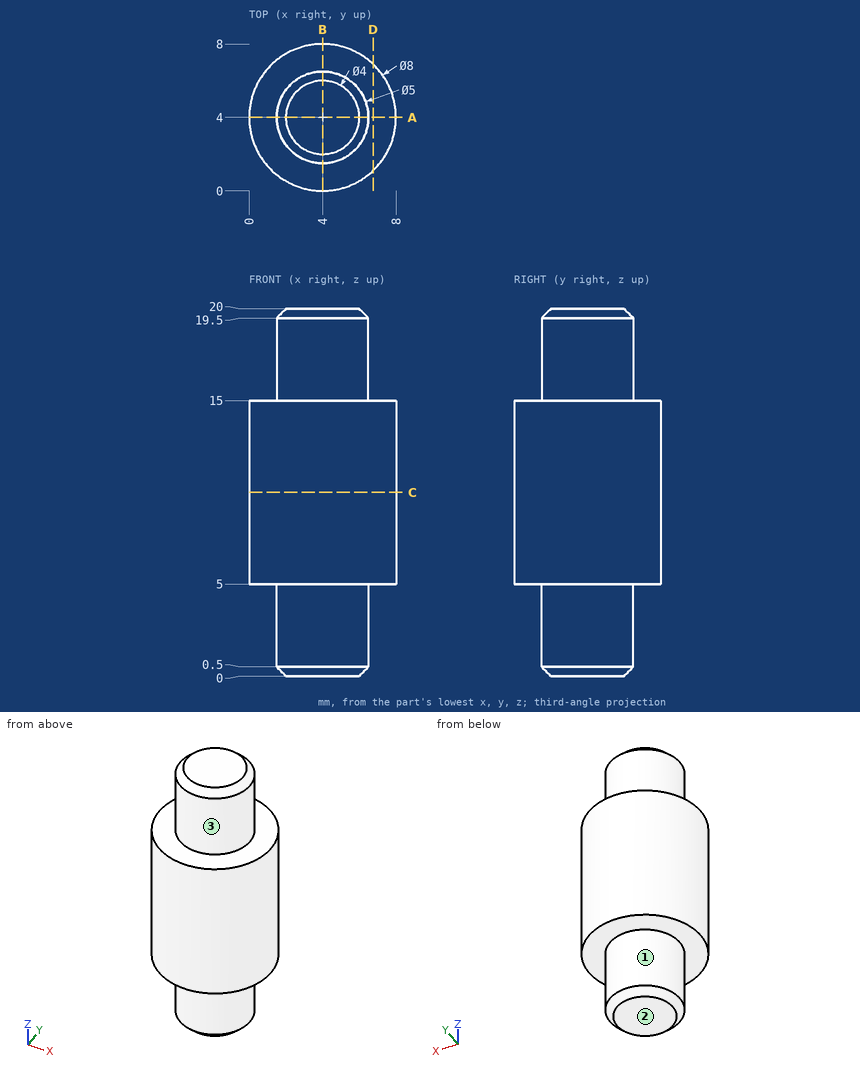
Design review of the part shown in the three views and the two pictorial views. Dimensions are in mm from the part's minimum x, y and z. A direction names the side the tool comes from. Round coordinates to 2 decimals unless told otherwise and drop trailing zeros. Loops run counter-clockwise (first coordinate to the right, second up) from the corner with the lowest first, then second, coordinate; pieces in that order, holes last. Notation, with made-up numbers: (-33, 32) - (-5, 32) arc R11 ccw to (-5, 43) - close; hole circle Ø10 at (51, 73.5). An arc over 180 degrees is marked (long way). Answer as CSV lines item,"result".
(1) Consider section D-D on x = 6.75. Give the boundary of the cut face in (y, z), then the cut area to 3 significant figures.
Checked values:
outline,"(1.1, 5) - (6.9, 5) - (6.9, 15) - (1.1, 15) - close"
area,"58.1 mm2"
(2) Wall thickness on line 1 (Z direction, x = 6.25, y = 5.25); line 2 (X direction, y = 5.5, z = 17); line 3 (Y direction, x = 5.5, z = 10.75): over which ranges is each line inside the solid? List them lowest first.
Checked values:
line 1,"z = 5 to 15"
line 2,"x = 2 to 6"
line 3,"y = 0.29 to 7.71"
(3) Consider section C-C on z = 10. Give the boundary of the cut face in (x, y), then the cut area to 3 significant figures.
Checked values:
outline,"circle Ø8 at (4, 4)"
area,"50.3 mm2"
(4) Tool access review of the marked faces 1, 2 and 3: name each direction out of +Z, -Z, +X, -X, +Y, -Y from which nothing blocks a thin tool from reaching the whole face with its end or side.
Checked values:
face 1,"-Z"
face 2,"-Z, +X, -X, +Y, -Y"
face 3,"+Z"
(5) Insertion check: P1, Ø1, axis at x = 5, y = 1.5, coming from the +Z side. The pin has a flat end and moves straight along its axis. Give the tip position at first contact, or say it passes through.
Checked values:
P1,"stops at z = 19.81"
(6) Consider section A-A on y = 4. Give the boundary of the cut face in (x, z), then the cut area to 4 significant figures.
Checked values:
outline,"(0, 5) - (1.5, 5) - (1.5, 0.5) - (2, 0) - (6, 0) - (6.5, 0.5) - (6.5, 5) - (8, 5) - (8, 15) - (6.5, 15) - (6.5, 19.5) - (6, 20) - (2, 20) - (1.5, 19.5) - (1.5, 15) - (0, 15) - close"
area,"129.5 mm2"
